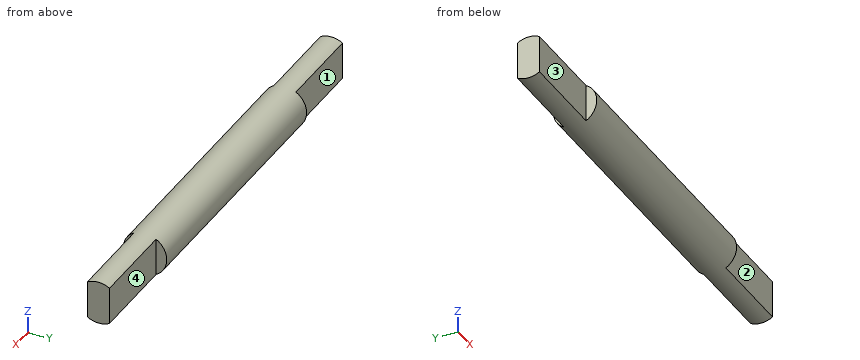
```python
from build123d import *

# Parameters (mm, degrees)
SKETCH1_R           = 2.45
BOSS_EXTRUDE1_DEPTH = 50
CUT_EXTRUDE1_DEPTH  = 10
CUT_EXTRUDE2_START  = -50
CUT_EXTRUDE2_DEPTH  = 10


with BuildPart() as part:
    # Sketch1 → Boss-Extrude1 (new body)
    with BuildSketch(Plane(origin=(0, 0, 0), x_dir=(0, 0, -1), z_dir=(1, 0, 0))):
        Circle(SKETCH1_R)
    extrude(amount=BOSS_EXTRUDE1_DEPTH)

    # Sketch2 → Cut-Extrude1 (cut)
    with BuildSketch(Plane(origin=(50, 0, 0), x_dir=(0, 0, -1), z_dir=(1, 0, 0))):
        with BuildLine():
            Line((-2.110088861, 1.245), (2.110088861, 1.245))
            ThreePointArc((2.110088861, 1.245), (0, 2.45), (-2.110088861, 1.245))
        make_face()
        with BuildLine():
            Line((-2.110088861, -1.245), (2.110088861, -1.245))
            ThreePointArc((2.110088861, -1.245), (0, -2.45), (-2.110088861, -1.245))
        make_face()
    extrude(amount=-CUT_EXTRUDE1_DEPTH, mode=Mode.SUBTRACT)

    # Sketch2<2> → Cut-Extrude2 (cut)
    with BuildSketch(Plane(origin=(50, 0, 0), x_dir=(0, 0, -1), z_dir=(1, 0, 0)).offset(CUT_EXTRUDE2_START)):
        with BuildLine():
            Line((-2.110088861, 1.245), (2.110088861, 1.245))
            ThreePointArc((2.110088861, 1.245), (0, 2.45), (-2.110088861, 1.245))
        make_face()
        with BuildLine():
            Line((-2.110088861, -1.245), (2.110088861, -1.245))
            ThreePointArc((2.110088861, -1.245), (0, -2.45), (-2.110088861, -1.245))
        make_face()
    extrude(amount=CUT_EXTRUDE2_DEPTH, mode=Mode.SUBTRACT)


solid = part.part
```
The listing builds one solid part. Answer for the finished solid, in the listing's coordinates (mm). Face numbers are marked on the shaded views. A direction names the side the tool comes from. Give positions to 0.01 mm unless a question says otherwise; leave off trailing zeros. Loops run counter-clockwise (first coordinate to the right, second up) from the corner with the lowest first, then second, coordinate; pieces in that order, holes last. Notation, with made-up numbers: M -12,76.25 L 30,76.25 A18 cw 30,88.25 Z; hole C 52.5,87 d7. An arc over 180 degrees is marked long. One line per item, written item: value.
Q1. Flat-ended cylindrical pins translate along their axes: P1, Ø2, axis at x = 18.5, z = 1.5, coming from the -Y side; P2, Ø1, axis at y = 2, z = -0.5, coming from the -X side; P3, Ø1.3, axis at x = 47, z = 0, coming from the +Y side (3 decimals). Find the tip coordinate at first contact, or state that the pin passes through.
Working result:
P1: stops at y = -2.4
P2: stops at x = 10
P3: stops at y = 1.245
Q2. Find the intervals of material crossed by line 1 (X direction, y = 1.45, z = -1.3); line 2 (Z direction, x = 2, y = 0.15); line 3 (Y direction, x = 3, z = 1.5) (3 decimals), in increasing order. Write a range as from..to.
Working result:
line 1: x = 10..40
line 2: z = -2.45..2.45
line 3: y = -1.245..1.245
Q3. A cutting plane is placed at B-B on x = 32.5. Determine the outline of the cut face in (y, z), then the cut area to 3 significant figures.
Working result:
outline: C 0,0 d4.9
area: 18.9 mm^2
Q4. A cutting plane is placed at C-C on y = 2. Determine the outline of the cut face in (x, z), then the cut area to 3 significant figures.
Working result:
outline: M 10,-1.42 L 40,-1.42 L 40,1.42 L 10,1.42 Z
area: 84.9 mm^2
Q5. A cutting plane is placed at D-D on x = 4. Determine the outline of the cut face in (y, z) (3 decimals), then the cut area to 3 significant figures.
Working result:
outline: M -1.245,-2.11 A2.45 ccw 1.245,-2.11 L 1.245,2.11 A2.45 ccw -1.245,2.11 Z
area: 11.7 mm^2
Q6. For the marked faces 1, 2, 3 and 4, determine the directions among +Z, -Z, +X, -X, +Y, -Y from which every point of the face is accessible in a straight line to the end or side of a thin tool.
Working result:
face 1: +Z, -Z, -X, +Y
face 2: +Z, -Z, +X, -Y
face 3: +Z, -Z, -X, -Y
face 4: +Z, -Z, +X, +Y
Q7. A cutting plane is placed at A-A on z = 0.45. Determine the outline of the cut face in (x, y) (3 decimals).
Working result:
outline: M 0,-1.245 L 10,-1.245 L 10,-2.408 L 40,-2.408 L 40,-1.245 L 50,-1.245 L 50,1.245 L 40,1.245 L 40,2.408 L 10,2.408 L 10,1.245 L 0,1.245 Z
